Geometry check sheet. Reference: the model listing, model coordinates, mm. Face numbers are marked on the shaded views. A direction names the side the tool comes from. Round coordinates to 2 decimals unless told otherwise and drop trailing zeros. Loops run counter-clockwise (first coordinate to the right, second up) from the corner with the lowest first, then second, coordinate; pieces in that order, holes last. Notation, with made-up numbers: M 67.25,61 L 114.25,61 A7 cw 114.25,73 Z; hole C 67,69.5 d10. An arc over 180 degrees is marked long. Write item = value, one per line.
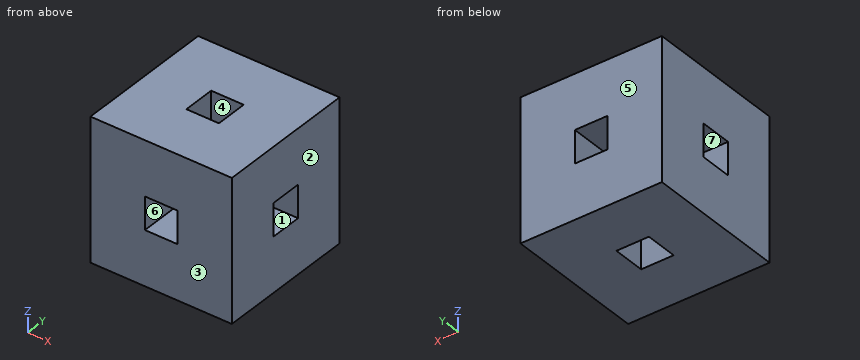
from build123d import *

# Parameters (mm, degrees)
F0_W     = 10
F0_H     = 10
F1_DEPTH = 10
F2_W     = 2.3
F2_H     = 2.3
F5_DEPTH = 10.001
F3_W     = 2.3
F3_H     = 2.3
F6_DEPTH = 10.001
F4_W     = 2.3
F4_H     = 2.3
F7_DEPTH = 10.001


with BuildPart() as f1:
    # F0 (on Top) → F1 (new body)
    with BuildSketch(Plane.XY):
        with Locations((-7.52488, 7.208158)):
            Rectangle(F0_W, F0_H)
    extrude(amount=F1_DEPTH)

    # F2 (on face) → F5 (cut, through all)
    with BuildSketch(Plane.XY.offset(10)):
        with Locations((-7.52488, 7.208158)):
            Rectangle(F2_W, F2_H)
    extrude(amount=-F5_DEPTH, mode=Mode.SUBTRACT)

    # F3 (on face) → F6 (cut, through all)
    with BuildSketch(Plane.XZ.offset(-2.208158)):
        with Locations((-7.52488, 5)):
            Rectangle(F3_W, F3_H)
    extrude(amount=-F6_DEPTH, mode=Mode.SUBTRACT)

    # F4 (on face) → F7 (cut, through all)
    with BuildSketch(Plane.YZ.offset(-2.52488)):
        with Locations((7.208158, 5)):
            Rectangle(F4_W, F4_H)
    extrude(amount=-F7_DEPTH, mode=Mode.SUBTRACT)


solid = f1.part
(1) Material ranges on line 1 along Z through (x, y) = (-7.5, 9.5); line 2 along X through (y, z) = (8.75, 5.25); line 3 along Y through (x, z) = (-5, 4.75), recorded low to high. Write a range as from..to.
Result set:
line_1 = 0..3.85, 6.15..10
line_2 = -12.52..-8.67, -6.37..-2.52
line_3 = 2.21..6.06, 8.36..12.21
(2) Tool access check on the marked faces 4, 5, 6 and 7. Record the directions out of +Z, -Z, +X, -X, +Y, -Y that give a thin tool (end or side, any length) a straight path to the whole face; none if there is none.
Result set:
face_4 = +Z, -Z
face_5 = +Z, -Z, +X, -X, +Y
face_6 = +Y, -Y
face_7 = +X, -X
(3) Sectioned sample at B-B on y = 10.5. Record the cut outline in (x, z).
Result set:
outline = M -12.52,0 L -2.52,0 L -2.52,10 L -12.52,10 Z; hole M -8.67,3.85 L -6.37,3.85 L -6.37,6.15 L -8.67,6.15 Z
(4) Sectioned sample at D-D on z = 8.25. Record the cut outline in (x, y).
Result set:
outline = M -12.52,2.21 L -2.52,2.21 L -2.52,12.21 L -12.52,12.21 Z; hole M -8.67,6.06 L -6.37,6.06 L -6.37,8.36 L -8.67,8.36 Z
(5) Release check for a two-part mould opening along Y. For the marked faces 1, 2 and 3 record: released by +Y, released by -Y, zero draft, split by the parting line, or undercut.
Result set:
face_1 = undercut
face_2 = zero draft
face_3 = released by -Y
(6) Sectioned sample at C-C on z = 6. Record the cut outline in (x, y), then the cut area to 3 significant figures.
Result set:
outline = M -12.52,2.21 L -8.67,2.21 L -8.67,6.06 L -12.52,6.06 Z; M -12.52,8.36 L -8.67,8.36 L -8.67,12.21 L -12.52,12.21 Z; M -6.37,2.21 L -2.52,2.21 L -2.52,6.06 L -6.37,6.06 Z; M -6.37,8.36 L -2.52,8.36 L -2.52,12.21 L -6.37,12.21 Z
area = 59.3 mm2
(7) Sectioned sample at A-A on x = -7.25. Record the cut outline in (y, z).
Result set:
outline = M 2.21,0 L 6.06,0 L 6.06,3.85 L 2.21,3.85 Z; M 2.21,6.15 L 6.06,6.15 L 6.06,10 L 2.21,10 Z; M 8.36,0 L 12.21,0 L 12.21,3.85 L 8.36,3.85 Z; M 8.36,6.15 L 12.21,6.15 L 12.21,10 L 8.36,10 Z
